```python
from build123d import *

# Parameters (mm, degrees)
F0_W     = 273.05
F0_H     = 114.3
F1_DEPTH = 19.05
F3_DEPTH = 25.4
F5_DEPTH = 25.4


with BuildPart() as f1:
    # F0 (on Front) → F1 (new body)
    with BuildSketch(Plane.XZ):
        with Locations((136.525, 57.15)):
            Rectangle(F0_W, F0_H)
    extrude(amount=F1_DEPTH)

    # F2 (on face) → F3 (cut)
    with BuildSketch(Plane.XZ.offset(19.05)):
        with BuildLine():
            ThreePointArc((72.8078575524, 38.1187458841), (75.3373142564, 44.2364484398), (76.2, 50.8))
            ThreePointArc((76.2, 50.8), (32.4977854296, 68.4121816315), (51.7756738724, 25.4187458841))
            Line((51.7756738724, 25.4187458841), (64.3298327923, 38.1187458841))
            Line((64.3298327923, 38.1187458841), (72.8078575524, 38.1187458841))
        make_face()
        with BuildLine():
            ThreePointArc((200.2421424476, 38.1187458841), (209.1205225089, 29.0565683295), (221.2743261276, 25.4187458841))
            Line((221.2743261276, 25.4187458841), (223.2256738724, 25.4187458841))
            Line((223.2256738724, 25.4187458841), (207.7043950558, 38.1187458841))
            Line((207.7043950558, 38.1187458841), (200.2421424476, 38.1187458841))
        make_face()
        with BuildLine():
            Line((223.2256738724, 25.4187458841), (221.2743261276, 25.4187458841))
            ThreePointArc((221.2743261276, 25.4187458841), (222.25, 25.4), (223.2256738724, 25.4187458841))
        make_face()
        with BuildLine():
            Line((64.3298327923, 38.1187458841), (51.7756738724, 25.4187458841))
            ThreePointArc((51.7756738724, 25.4187458841), (63.9294774911, 29.0565683295), (72.8078575524, 38.1187458841))
            Line((72.8078575524, 38.1187458841), (64.3298327923, 38.1187458841))
        make_face()
        with BuildLine():
            ThreePointArc((247.65, 50.8), (215.6864484398, 75.3373142564), (200.2421424476, 38.1187458841))
            Line((200.2421424476, 38.1187458841), (207.7043950558, 38.1187458841))
            Line((207.7043950558, 38.1187458841), (223.2256738724, 25.4187458841))
            ThreePointArc((223.2256738724, 25.4187458841), (240.5522145704, 33.1878183685), (247.65, 50.8))
        make_face()
        with BuildLine():
            Line((100.33, 44.45), (151.0539650917, 44.45))
            Line((151.0539650917, 44.45), (172.72, 44.45))
            ThreePointArc((172.72, 44.45), (180.802230509, 47.797769491), (184.15, 55.88))
            Line((184.15, 55.88), (184.15, 114.3))
            Line((184.15, 114.3), (88.9, 114.3))
            Line((88.9, 114.3), (88.9, 55.88))
            ThreePointArc((88.9, 55.88), (92.247769491, 47.797769491), (100.33, 44.45))
        make_face()
    extrude(amount=-F3_DEPTH, mode=Mode.SUBTRACT)

    # F4 (on face) → F5 (cut)
    with BuildSketch(Plane.XZ.offset(19.05)):
        with BuildLine():
            Line((172.72, 44.45), (147.32, 44.45))
            Line((147.32, 44.45), (147.32, 38.1542206768))
            Line((147.32, 38.1542206768), (72.8282606056, 38.1542206768))
            ThreePointArc((72.8282606056, 38.1542206768), (64.2384219855, 29.2461415394), (52.4587557079, 25.4542206768))
            Line((52.4587557079, 25.4542206768), (220.5912442921, 25.4542206768))
            ThreePointArc((220.5912442921, 25.4542206768), (208.8115780145, 29.2461415394), (200.2217393944, 38.1542206768))
            Line((200.2217393944, 38.1542206768), (172.72, 38.1542206768))
            Line((172.72, 38.1542206768), (172.72, 44.45))
        make_face()
    extrude(amount=-F5_DEPTH, mode=Mode.SUBTRACT)


solid = f1.part
```
Read the model definition and answer for the solid it produces. Units are mm, in the model's axes. A direction names the side the tool comes from. Give positions to 0.01 mm unless a question says otherwise; leave off trailing zeros. Loops run counter-clockwise (first coordinate to the right, second up) from the corner with the lowest first, then second, coordinate; pieces in that order, holes last.
Item 1: The mould has two halves that part along Z. Classify faces 1 (the flat face through (111, -10, 38.154)), 2 (the flat face through (273.05, -9, 56)), 3 (the flat face through (228, -9, 114.3)): released by +Z, released by -Z, zero draft, split by the parting line, or undercut.
Item 2: The part is cut by section A-A (x = 120). Write down the section's boundary in (y, z), and give its area (3 significant figures).
Item 3: Each of these flat-tipped pins is pushed along its axis until it touches: pin 1 Ø5.5 at (x, y) = (166, -14) entering from +Z; pin 2 Ø9.5 at (x, y) = (129, -7) entering from +Z. Where does it stop, or does it pass through?
Item 4: For faces 4 (the flat face through (0, -9, 56)), 5 (the cylindrical face through (92.159, -9.658, 47.887)), 6 (the flat face through (187, -10, 38.154)), determine the directions among +Z, -Z, +X, -X, +Y, -Y from which every point of the face is accessible in a straight line to the end or side of a thin tool.
Item 5: The part is cut by section C-C (y = -11). Write down the section's boundary in (x, z), and give its area (3 significant figures).
Item 6: Find the intervals of material crossed by line 1 along X through (y, z) = (-2, 73); line 2 along X through (y, z) = (-7.25, 50.8); line 3 along X through (y, z) = (-18, 100), in increasing order.
Item 7: The part is cut by section B-B (z = 41.5). Write down the section's boundary in (x, y).
Item 8: The part is cut by section D-D (x = 190). Write down the section's boundary in (y, z), and give its area (3 significant figures).
Taken from the geometry:
1. face 1: undercut
1. face 2: zero draft
1. face 3: released by +Z
2. outline: (-19.05, 0) - (0, 0) - (0, 25.45) - (-19.05, 25.45) - close; (-19.05, 38.15) - (0, 38.15) - (0, 44.45) - (-19.05, 44.45) - close
2. area: 605 mm2
3. pin 1: stops at z = 25.45
3. pin 2: stops at z = 44.45
4. face 4: +Z, -Z, -X, +Y, -Y
4. face 5: +Z, +Y, -Y
4. face 6: +Y, -Y
5. outline: (0, 0) - (273.05, 0) - (273.05, 114.3) - (184.15, 114.3) - (184.15, 55.88) arc R11.43 cw to (172.72, 44.45) - (172.72, 38.15) - (200.22, 38.15) arc R25.4 cw (long way) to (220.59, 25.45) - (52.46, 25.45) arc R25.4 cw (long way) to (72.83, 38.15) - (147.32, 38.15) - (147.32, 44.45) - (100.33, 44.45) arc R11.43 cw to (88.9, 55.88) - (88.9, 114.3) - (0, 114.3) - close
5. area: 18,600 mm2
6. line 1: x = 0 to 38.46, 63.14 to 88.9, 184.15 to 209.91, 234.59 to 273.05
6. line 2: x = 0 to 25.4, 76.2 to 90.09, 182.96 to 196.85, 247.65 to 273.05
6. line 3: x = 0 to 88.9, 184.15 to 273.05
7. outline: (0, -19.05) - (27.16, -19.05) - (27.16, 0) - (0, 0) - close; (74.44, -19.05) - (147.32, -19.05) - (147.32, 0) - (74.44, 0) - close; (172.72, -19.05) - (198.61, -19.05) - (198.61, 0) - (172.72, 0) - close; (245.89, -19.05) - (273.05, -19.05) - (273.05, 0) - (245.89, 0) - close
8. outline: (-19.05, 0) - (0, 0) - (0, 25.45) - (-19.05, 25.45) - close; (-19.05, 38.15) - (0, 38.15) - (0, 114.3) - (-19.05, 114.3) - close
8. area: 1,940 mm2
